Solid Edge part; units mm, degrees
sketch "Sketch1" plane through (0, 0, 0) normal (0, 0, 1) x (1, 0, 0)
  circle A0 centre (0, 0) radius 6.4452
extrude "Protrusion1" add sketch "Sketch1" along normal blind 3.048
sketch "Sketch2" plane through (0, 0, 0) normal (0, 0, -1) x (1, 0, 0)
  circle A0 centre (0, 0) radius 2.413
extrude "Protrusion2" add sketch "Sketch2" along normal blind 25.4
sketch "Sketch3" plane through (0, 0, -25.4) normal (0, 0, -1) x (1, 0, 0)
  circle A0 centre (0, 0) radius 2.4127
extrude "Cutout1" cut sketch "Sketch3" against normal blind 25.3746 flip side to cut
sketch "Sketch4" plane through (0, 0, 3.048) normal (0, 0, 1) x (1, 0, 0)
  line L0 (-5.0784, 3.9688) -> (5.0784, 3.9688)
extrude "Cutout2" cut sketch "Sketch4" against normal up to next material side at (0, 4.0188, 3.048)
sketch "Sketch5" plane through (0, 0, 0) normal (1, 0, 0) x (0, 1, 0)
  line L0 (-0.7937, -25.4) -> (-2.4127, -22.5958)
revolve "RevolvedCutout1" cut sketch "Sketch5" angle 360 about axis through (0, 0, -14.7796) along (0, 0, 1) material side at (0, -1.6465, -24.0229)
pattern_circular "Pattern1" count 6 over 360 about axis through (0, 0, 3.048) along (0, 0, 1) of "Cutout2"
properties part number "24100703"
Check sheet for the modelled part. Datum: model origin and axes. Units: mm. A direction names the side the tool comes from. Give positions to 0.01 mm unless a question says otherwise; leave off trailing zeros. Order: outer loops, then holes, each group sorted by start corner. A loop starts at its lowest first (then second) coordinate and runs counter-clockwise, first axis right, second up. Notation, with made-up numbers: M 58,-2 L 115,-2 A31 ccw 115,36 Z; hole C 32.25,51 d9. An arc over 180 degrees is marked long. Answer as CSV lines item,"result". Start each with the question number.
Item 1: Cross-section at A-A on z = 1. Enter the section's corners in (x, y).
Item 2: Thickness scan on line 1 (Z direction, x = -1, y = 3); line 2 (Y direction, x = 0, z = -17); line 3 (X direction, y = -1.75, z = -17.75). Record the ranges inside material, lowest first. Write a range as [from, to].
Item 3: Cross-section at D-D on x = -3.25. Enter the section's corners in (y, z).
Item 4: Gauge pin test, flat ends, axial feed: P1, Ø1, axis at y = -1, z = -17.5, coming from the +X side; P2, Ø4, axis at x = -2.5, z = -21.5, coming from the +Y side; P3, Ø2, axis at x = 2, y = -2, coming from the -Z side. Record the tip position at first contact, or that the pin passes through.
Item 5: Tool access check on faces 1 (the face through (0, 3.969, 2)), 2 (the face through (-0.314, -2.392, -11.469)). Record the directions out of +Z, -Z, +X, -X, +Y, -Y that give a thin tool (end or side, any length) a straight path to the whole face; none if there is none.
Item 6: Cross-section at C-C on y = -2.75. Enter the section's corners in (x, z).
Established:
1,outline,"M -4.58,0 L -2.29,-3.97 L 2.29,-3.97 L 4.58,0 L 2.29,3.97 L -2.29,3.97 Z"
2,line 1,"z = [0, 3.05]"
2,line 2,"y = [-2.41, 2.41]"
2,line 3,"x = [-1.66, 1.66]"
3,outline,"M -2.31,0 L 2.31,0 L 2.31,3.05 L -2.31,3.05 Z"
4,P1,"stops at x = 2.36"
4,P2,"stops at y = 2.36"
4,P3,"stops at z = -23.61"
5,face 1,"+Z, -Z, +X, -X, +Y"
5,face 2,"-Z"
6,outline,"M -3,0 L 3,0 L 3,3.05 L -3,3.05 Z"
